The model under review builds one solid part; all positions refer to its coordinate system, in mm. A direction names the side the tool comes from. Give positions to 0.01 mm unless a question says otherwise; leave off trailing zeros. Loops run counter-clockwise (first coordinate to the right, second up) from the corner with the lowest first, then second, coordinate; pieces in that order, holes last. Notation, with made-up numbers: (26, 54) - (54, 54) arc R18 ccw to (54, 80) - close; hole circle Ø10 at (68.25, -2). An arc over 180 degrees is marked (long way). Answer as a JSON object with one key per item and string values.
from build123d import *

# Parameters (mm, degrees)
SKETCH1_W           = 170
SKETCH1_H           = 60
BOSS_EXTRUDE1_DEPTH = 20
FILLET1_R           = 5
BOSS_EXTRUDE2_DEPTH = 42
SKETCH5_R           = 15
BOSS_EXTRUDE3_DEPTH = 18
SKETCH6_R           = 10
CUT_EXTRUDE1_DEPTH  = 28
SKETCH7_W           = 40
SKETCH7_H           = 131.983318458
CUT_EXTRUDE2_DEPTH  = 10
FILLET5_R           = 3
SKETCH8_R           = 6.5
CUT_EXTRUDE3_DEPTH  = 20
SKETCH9_R           = 4
CUT_EXTRUDE4_DEPTH  = 60


with BuildPart() as part:
    # Sketch1 → Boss-Extrude1 (new body)
    with BuildSketch(Plane(origin=(0, 0, 0), x_dir=(1, 0, 0), z_dir=(0, 1, 0))):
        Rectangle(SKETCH1_W, SKETCH1_H)
    extrude(amount=BOSS_EXTRUDE1_DEPTH)

    # Fillet1
    fillet1_edges = [part.edges().sort_by_distance(p)[0] for p in [
        (-85, 10, -30),
        (85, 10, -30),
        (85, 10, 30),
        (-85, 10, 30),
    ]]
    fillet(fillet1_edges, radius=FILLET1_R)

    # Sketch4 → Boss-Extrude2 (add)
    with BuildSketch(Plane(origin=(0, 0, 12), x_dir=(-1, 0, 0), z_dir=(0, 0, -1))):
        with BuildLine():
            Line((48.849351026, 20), (58.849351026, 20))
            Line((58.849351026, 20), (58.849351026, 60))
            ThreePointArc((58.849351026, 60), (49.414627953, 93.726843908), (23.849351026, 117.662812973))
            Line((23.849351026, 117.662812973), (23.849351026, 138.983318458))
            ThreePointArc((23.849351026, 138.983318458), (22.970671369, 141.104638801), (20.849351026, 141.983318458))
            Line((20.849351026, 141.983318458), (-33.150648974, 141.983318458))
            ThreePointArc((-33.150648974, 141.983318458), (-35.271969318, 141.104638801), (-36.150648974, 138.983318458))
            Line((-36.150648974, 138.983318458), (-36.150648974, 88))
            ThreePointArc((-36.150648974, 88), (-35.271969318, 85.878679656), (-33.150648974, 85))
            Line((-33.150648974, 85), (14.083425542, 85))
            ThreePointArc((14.083425542, 85), (16.204745885, 84.121320344), (17.083425542, 82))
            Line((17.083425542, 82), (17.083425542, 45))
            Line((17.083425542, 45), (-5.824853809, 20))
            Line((-5.824853809, 20), (23.849351026, 20))
            Line((23.849351026, 20), (23.849351026, 95.707142143))
            ThreePointArc((23.849351026, 95.707142143), (26.912859353, 100.316914371), (32.349351026, 99.277856357))
            ThreePointArc((32.349351026, 99.277856357), (44.556845541, 81.301408404), (48.849351026, 60))
            Line((48.849351026, 60), (48.849351026, 20))
        make_face()
        Polygon((-36.150648974, 20), (-5.824853809, 20), (-28.733133159, 45), (-36.150648974, 45), align=None)
    extrude(amount=BOSS_EXTRUDE2_DEPTH)

    # Sketch5 → Boss-Extrude3 (add)
    with BuildSketch(Plane(origin=(0, 141.983318458, 0), x_dir=(1, 0, 0), z_dir=(0, 1, 0))):
        with Locations((6.150648974, 9)):
            Circle(SKETCH5_R)
    extrude(amount=BOSS_EXTRUDE3_DEPTH)

    # Sketch6 → Cut-Extrude1 (cut)
    with BuildSketch(Plane(origin=(0, 159.983318458, 0), x_dir=(1, 0, 0), z_dir=(0, 1, 0))):
        with Locations((6.150648974, 9)):
            Circle(SKETCH6_R)
    extrude(amount=-CUT_EXTRUDE1_DEPTH, mode=Mode.SUBTRACT)

    # Sketch7 → Cut-Extrude2 (cut, symmetric)
    with BuildSketch(Plane(origin=(0, 0, -9), x_dir=(-1, 0, 0), z_dir=(0, 0, -1))):
        with Locations((-6.150648974, 65.991659229)):
            Rectangle(SKETCH7_W, SKETCH7_H)
    extrude(amount=CUT_EXTRUDE2_DEPTH, both=True, mode=Mode.SUBTRACT)

    # Fillet5
    fillet5_edges = [part.edges().sort_by_distance(p)[0] for p in [
        (36.150648974, 20, -9),
        (-23.849351026, 20, -9),
        (-48.849351026, 20, -9),
        (-53.849351026, 20, 12),
        (-58.849351026, 20, -9),
    ]]
    fillet(fillet5_edges, radius=FILLET5_R)

    # Sketch8 → Cut-Extrude3 (cut)
    with BuildSketch(Plane(origin=(0, 20, 0), x_dir=(1, 0, 0), z_dir=(0, 1, 0))):
        with Locations((-70, 0)):
            Circle(SKETCH8_R)
        with Locations((70, 0)):
            Circle(SKETCH8_R)
    extrude(amount=-CUT_EXTRUDE3_DEPTH, mode=Mode.SUBTRACT)

    # Sketch9 → Cut-Extrude4 (cut)
    with BuildSketch(Plane(origin=(36.150648974, 0, 0), x_dir=(0, 0, -1), z_dir=(1, 0, 0))):
        with Locations((10, 124.983318458)):
            Circle(SKETCH9_R)
    extrude(amount=-CUT_EXTRUDE4_DEPTH, mode=Mode.SUBTRACT)


solid = part.part
Q1. Consider section A-A, the plane x = -70. State the section outline as (y, z) points, plus the area to 3 significant figures.
Results:
{"outline": "(0, -30) - (20, -30) - (20, -6.5) - (0, -6.5) - close; (0, 6.5) - (20, 6.5) - (20, 30) - (0, 30) - close", "area": "940 mm^2"}
Q2. Consider section B-B, the plane y = 25.5. State the section outline as (x, z) points, plus the area to 3 significant figures.
Results:
{"outline": "(-58.85, -30) - (-48.85, -30) - (-48.85, 12) - (-58.85, 12) - close; (-23.85, -30) - (0.79, -30) - (0.79, -19) - (-13.85, -19) - (-13.85, 1) - (0.79, 1) - (0.79, 12) - (-23.85, 12) - close; (10.86, -30) - (36.15, -30) - (36.15, 12) - (10.86, 12) - (10.86, 1) - (26.15, 1) - (26.15, -19) - (10.86, -19) - close", "area": "1,920 mm^2"}
Q3. To check wall thickness, follow probe 1 along X at (y, z) = (31, -13.5); probe 2 along X at (y, z) = (5.5, 0); probe 3 along Y at (x, z) = (33, -10). State the ranges of each line that lie inside material, in increasing order. Write a range as [from, to].
Results:
{"probe 1": "x = [-58.85, -48.85], [-23.85, -13.85], [26.15, 36.15]", "probe 2": "x = [-85, -76.5], [-63.5, -13.85], [26.15, 63.5], [76.5, 85]", "probe 3": "y = [0, 45], [85, 120.98], [128.98, 141.98]"}
Q4. For faces 1 (the face through (36.151, 34, -9)), 2 (the face through (-58.849, 41, -9)), 3 (the face through (-23.849, 59, -9)), list the 3-axis set-ups (+Z, -Z, +X, -X, +Y, -Y) from which the entire face can be reached by the end or side of a thin tool; tool diameter is ignored.
Results:
{"face 1": "+Z, -Z, +X, +Y", "face 2": "+Z, -Z, -X, +Y", "face 3": "+Z, -Z"}
Q5. Consider section D-D, the plane z = -9. State how many separate pieces and enclosed holes the cut face has, plus the area to 3 significant figures.
Results:
{"separate pieces": "5", "enclosed holes": "1", "area": "5,780 mm^2"}
Q6. Clearance check with flat-ended pins moving along their axes: pin 1 Ø10.5 at (x, z) = (70, 0) entering from +Y; pin 2 Ø12 at (x, y) = (-0.5, 110) entering from +Z; pin 3 Ø2 at (y, z) = (70.5, -21.5) entering from -X; pin 4 Ø13 at (y, z) = (124.98, -10) entering from +X. State where each tip first meets the part, or that it passes through.
Results:
{"pin 1": "passes through", "pin 2": "stops at z = 12", "pin 3": "stops at x = -58.15", "pin 4": "stops at x = 36.15"}
Q7. The part is to be moulded in two halves that separate along X. For faces 4 (the face through (-44.44, 81.58, -8.71)), 5 (the face through (10, 85, 5)), 6 (the face through (-13.849, 20, -9)), 7 (the face through (-84, 10, -28)), say which applies: +X half, -X half, draft (parallel to the pull), parting line (faces both ways), or undercut.
Results:
{"face 4": "undercut", "face 5": "draft", "face 6": "undercut", "face 7": "-X half"}
